Geometry check sheet. Reference: the model listing, model coordinates, mm. Face numbers are marked on the shaded views. Round coordinates to 2 decimals unless told otherwise and drop trailing zeros. Order: outer loops, then holes, each group sorted by start corner. A loop starts at its lowest first (then second) coordinate and runs counter-clockwise, first axis right, second up. Notation, with made-up numbers: (88, 60) -> (112, 60) arc R14 ccw to (112, 79) -> close; hole circle Ø1 at (77, 46). An arc over 180 degrees is marked (long way). Answer as a JSON object with one key per item and string values. Group by question number.
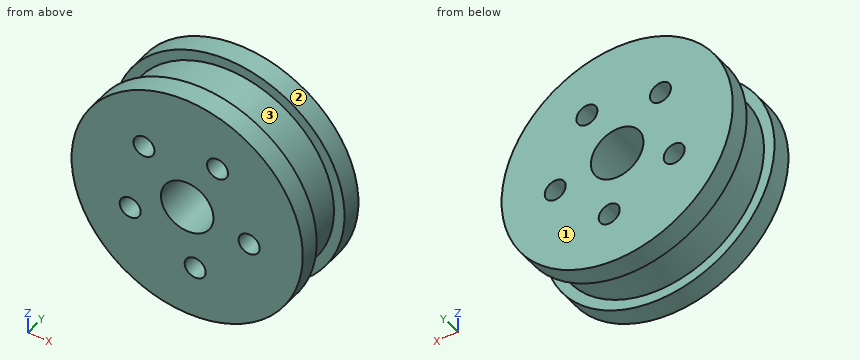
from build123d import *

# Parameters (mm, degrees)
SKETCH4_R          = 3.175
CUT_EXTRUDE3_DEPTH = 33.848593577
SKETCH6_R          = 1.27
CUT_EXTRUDE5_DEPTH = 33.848593577


with BuildPart() as part:
    # Sketch1 → Revolve1 (revolve)
    with BuildSketch(Plane.XY, mode=Mode.PRIVATE) as revolve1_sk:
        Polygon((0, 0), (0, 2.54), (13.97, 2.54), (13.97, -7.62), (0, -7.62), (0, -5.08), (1.27, -5.08), (1.27, 0), align=None)
    revolve(revolve1_sk.sketch.rotate(Axis((13.97, -7.62, 0), (0, 1, 0)), 270), axis=Axis((13.97, -7.62, 0), (0, 1, 0)))

    # Sketch4 → Cut-Extrude3 (cut, through all)
    with BuildSketch(Plane(origin=(0, 2.54, 0), x_dir=(1, 0, 0), z_dir=(0, 1, 0))):
        with Locations(Location((13.97, 0, 0), (0, 0, 270))):
            Circle(SKETCH4_R)
    extrude(amount=-CUT_EXTRUDE3_DEPTH, mode=Mode.SUBTRACT)

    # Sketch6 → Cut-Extrude5 (cut, through all)
    with BuildSketch(Plane(origin=(0, 2.54, 0), x_dir=(1, 0, 0), z_dir=(0, 1, 0))):
        with Locations(Location((7.079305779, 3.253111304, 0), (0, 0, 270))):
            Circle(SKETCH6_R)
        with Locations(Location((14.934551087, 7.558706318, 0), (0, 0, 270))):
            Circle(SKETCH6_R)
        with Locations(Location((21.456819576, 1.418426111, 0), (0, 0, 270))):
            Circle(SKETCH6_R)
        with Locations(Location((17.632557879, -6.682070771, 0), (0, 0, 270))):
            Circle(SKETCH6_R)
        with Locations(Location((8.746765678, -5.548172963, 0), (0, 0, 270))):
            Circle(SKETCH6_R)
    extrude(amount=-CUT_EXTRUDE5_DEPTH, mode=Mode.SUBTRACT)


solid = part.part
Item 1: Sectioned sample at D-D, the plane x = 2. Enter the section's corners in (y, z), then the cut area to 3 significant figures.
Item 2: Mould release check, pull along Y, two halves, no side actions. Record for the marked faces 1, 2 and 3: pulls with the +Y half, pulls with the -Y half, needs draft (parallel to the pull), parting line crosses it, or undercut.
Item 3: Thickness scan on L1, parallel to Y at x = 4.25, z = 8.5; L2, parallel to Z at x = 16.5, y = 2.25; L3, parallel to X at y = -5, z = 6.5. Record the ranges inside material, lowest first.
Item 4: Depth check by flat-ended pin: pin 1 Ø3 at (x, y) = (24, 0.5) entering from +Z; pin 2 Ø6 at (y, z) = (0, 5) entering from +X; pin 3 Ø3 at (x, z) = (21.46, -1.42) entering from +Y. Enter the tip coordinate at first touch or a pass-through.
Item 5: Sectioned sample at C-C, the plane z = -5.25. Enter the section's corners in (x, y).
Item 6: Sectioned sample at B-B, the plane y = -3.5. Enter the section's corners in (x, z) (3 decimals), then the cut area to 3 significant figures.
Item 7: Sectioned sample at A-A, the plane x = 13. Enter the section's corners in (y, z).
Result:
{
 "1": {"outline": "(-7.62, -7.2) -> (-5.08, -7.2) -> (-5.08, -4.24) -> (0, -4.24) -> (0, -7.2) -> (2.54, -7.2) -> (2.54, 7.2) -> (0, 7.2) -> (0, 4.24) -> (-5.08, 4.24) -> (-5.08, 7.2) -> (-7.62, 7.2) -> close", "area": "116 mm2"},
 "2": {"face 1": "pulls with the +Y half", "face 2": "needs draft", "face 3": "undercut"},
 "3": {"L1": "y = -7.62 to -5.08, 0 to 2.54", "L2": "z = -13.74 to -1.92, 1.92 to 6.11, 7.26 to 13.74", "L3": "x = 3.06 to 7.91, 9.59 to 16.38, 18.89 to 24.88"},
 "4": {"pin 1": "stops at z = 11.06", "pin 2": "stops at x = 27.8", "pin 3": "stops at y = 2.54"},
 "5": {"outline": "(1.02, -7.62) -> (26.92, -7.62) -> (26.92, -5.08) -> (25.53, -5.08) -> (25.53, 0) -> (26.92, 0) -> (26.92, 2.54) -> (1.02, 2.54) -> (1.02, 0) -> (2.41, 0) -> (2.41, -5.08) -> (1.02, -5.08) -> close"},
 "6": {"outline": "circle Ø25.4 at (13.97, 0); hole circle Ø2.54 at (7.079, -3.253); hole circle Ø2.54 at (8.747, 5.548); hole circle Ø6.35 at (13.97, 0); hole circle Ø2.54 at (14.935, -7.559); hole circle Ø2.54 at (17.633, 6.682); hole circle Ø2.54 at (21.457, -1.418)", "area": "450 mm2"},
 "7": {"outline": "(-7.62, -13.94) -> (-5.08, -13.94) -> (-5.08, -12.66) -> (0, -12.66) -> (0, -13.94) -> (2.54, -13.94) -> (2.54, -3.02) -> (-7.62, -3.02) -> close; (-7.62, 3.02) -> (2.54, 3.02) -> (2.54, 13.94) -> (0, 13.94) -> (0, 12.66) -> (-5.08, 12.66) -> (-5.08, 13.94) -> (-7.62, 13.94) -> close"}
}
